```python
from build123d import *

# Parameters (mm, degrees)
SKETCH_1_R               = 20.5
EXTRUDE_1_DEPTH          = 5
HOLE_WIZARD_M5_1_D       = 5.3
HOLE_WIZARD_M5_2_D       = 5.3
HOLE_WIZARD_M5_2_DEPTH   = 5
CUT_EXTRUDE_1_DEPTH      = 2.5
HOLE_WIZARD_2_0_2_1_D    = 2
PATTERN_CIRCULAR_1_COUNT = 2


with BuildPart() as part:
    # 스케치1 → 보스-돌출1 (new, symmetric)
    with BuildSketch(Plane.XY):
        Circle(SKETCH_1_R)
    extrude(amount=EXTRUDE_1_DEPTH, both=True)

    # M5 여유 구멍1 (through all)
    with Locations(Plane.XY.offset(5)):
        with Locations((0, 0)):
            Hole(HOLE_WIZARD_M5_1_D / 2)

    # M5 여유 구멍2
    with Locations(Plane(origin=(0, 0, -5), x_dir=(-1, 0, 0), z_dir=(0, 0, -1))):
        with Locations((12.5, 0)):
            hole_wizard_m5_2 = Hole(HOLE_WIZARD_M5_2_D / 2, depth=HOLE_WIZARD_M5_2_DEPTH)

    # 대칭 복사1: M5 여유 구멍2 across plane
    add(hole_wizard_m5_2.mirror(Plane(origin=(0, 0, 0), x_dir=(0, 0, 1), z_dir=(1, 0, 0))), mode=Mode.SUBTRACT)

    # 스케치6 → 컷-돌출1 (cut)
    with BuildSketch(Plane.XY.offset(5)):
        with BuildLine():
            ThreePointArc((7.778174593, 7.778174593), (0, 11), (-7.778174593, 7.778174593))
            ThreePointArc((-7.778174593, 7.778174593), (-7.778174593, 3.535533906), (-3.535533906, 3.535533906))
            ThreePointArc((-3.535533906, 3.535533906), (0, 5), (3.535533906, 3.535533906))
            ThreePointArc((3.535533906, 3.535533906), (7.778174593, 3.535533906), (7.778174593, 7.778174593))
        make_face()
    cut_extrude_1 = extrude(amount=-CUT_EXTRUDE_1_DEPTH, mode=Mode.SUBTRACT)

    # Ø2.0 (2) 지름 구멍1 (through all)
    with Locations(Plane.XY.offset(2.5)):
        with Locations((0, 8)):
            hole_wizard_2_0_2_1 = Hole(HOLE_WIZARD_2_0_2_1_D / 2)

    # 원형 패턴1: 컷-돌출1, Ø2.0 (2) 지름 구멍1 ×2 about axis
    pattern_circular_1_axis = Axis((0, 0, 0), (0, 0, 1))
    add([cut_extrude_1.rotate(pattern_circular_1_axis, i * 360 / PATTERN_CIRCULAR_1_COUNT) for i in range(1, PATTERN_CIRCULAR_1_COUNT)], mode=Mode.SUBTRACT)
    add([hole_wizard_2_0_2_1.rotate(pattern_circular_1_axis, i * 360 / PATTERN_CIRCULAR_1_COUNT) for i in range(1, PATTERN_CIRCULAR_1_COUNT)], mode=Mode.SUBTRACT)


solid = part.part
```
The model under review builds one solid part; all positions refer to its coordinate system, in mm. A direction names the side the tool comes from. Round coordinates to 2 decimals unless told otherwise and drop trailing zeros. Order: outer loops, then holes, each group sorted by start corner. A loop starts at its lowest first (then second) coordinate and runs counter-clockwise, first axis right, second up. Notation, with made-up numbers: M 25.5,88 L 36.5,88 A19 cw 36.5,106 Z; hole C 13,0.5 d9. An arc over 180 degrees is marked long. Use a Markdown table: item, result.
1) Consider section B-B (z = -3.75). Write out the cut boundary in (x, y), then the cut area to 3 significant figures.
Report:
| item | result |
|---|---|
| outline | C 0,0 d41; hole C -12.5,0 d5.3; hole C 0,0 d5.3; hole C 0,-8 d2; hole C 0,8 d2; hole C 12.5,0 d5.3 |
| area | 1,250 mm^2 |
2) Consider section A-A (x = 0). Write out the cut boundary in (y, z).
Report:
| item | result |
|---|---|
| outline | M -20.5,-5 L -9,-5 L -9,2.5 L -11,2.5 L -11,5 L -20.5,5 Z; M -7,-5 L -2.65,-5 L -2.65,5 L -5,5 L -5,2.5 L -7,2.5 Z; M 2.65,-5 L 7,-5 L 7,2.5 L 5,2.5 L 5,5 L 2.65,5 Z; M 9,-5 L 20.5,-5 L 20.5,5 L 11,5 L 11,2.5 L 9,2.5 Z |
3) Wall thickness on line 1 along Y through (x, z) = (0, -2); line 2 along Y through (x, z) = (-7.5, 4); line 3 along Z through (x, y) = (-7, -6.5): over which ranges is each line inside the solid? List them lowest first. Write a range as [from, to].
Report:
| item | result |
|---|---|
| line 1 | [-20.5, -9], [-7, -2.65], [2.65, 7], [9, 20.5] |
| line 2 | [-19.08, -8.05], [-3.29, 3.29], [8.05, 19.08] |
| line 3 | [-5, 2.5] |
4) Insertion check: pin 1 (2.5 mm diameter, centred on x = -13.5, y = -0.5, fed in from -Z); pin 2 (6 mm diameter, centred on y = -11.5, z = 1.5, fed in from +X); pin 3 (1 mm diameter, centred on x = 7.5, z = -1, fed in from -Y); pin 4 (5 mm diameter, centred on x = 0, y = 0, fed in from -Z). Each pin has a flat end and moves straight along its axis. Give the tip position at first contact, or say it passes through.
Report:
| item | result |
|---|---|
| pin 1 | z = 0 |
| pin 2 | x = 18.65 |
| pin 3 | y = -19.27 |
| pin 4 | through |
5) Tool access review of faces 1 (the face through (-10.05, -1.01, -2.46)), 2 (the face through (0, -5, 4)), 3 (the face through (0, -9, -1)): name each direction out of +Z, -Z, +X, -X, +Y, -Y from which nothing blocks a thin tool from reaching the whole face with its end or side.
Report:
| item | result |
|---|---|
| face 1 | -Z |
| face 2 | +Z |
| face 3 | +Z, -Z |
6) Draft analysis for pull direction Y (two halves, no side actions). For faces 4 (the face through (13, 0, 0)), 5 (the face through (-4.444, -20.013, 0.07)), 6 (the face through (4, 0, -5)), state which applies: released by +Y, released by -Y, zero draft, split by the parting line, or undercut.
Report:
| item | result |
|---|---|
| face 4 | undercut |
| face 5 | split by the parting line |
| face 6 | zero draft |
7) Consider section C-C (y = -2). Write out the cut boundary in (x, z).
Report:
| item | result |
|---|---|
| outline | M -20.4,-5 L -14.24,-5 L -14.24,0 L -10.76,0 L -10.76,-5 L -1.74,-5 L -1.74,5 L -20.4,5 Z; M 1.74,-5 L 10.76,-5 L 10.76,0 L 14.24,0 L 14.24,-5 L 20.4,-5 L 20.4,5 L 1.74,5 Z |
8) Consider section D-D (z = 3.25). Write out the cut boundary in (x, y).
Report:
| item | result |
|---|---|
| outline | C 0,0 d41; hole M -7.78,-7.78 A11 ccw 7.78,-7.78 A3 ccw 3.54,-3.54 A5 cw -3.54,-3.54 A3 ccw Z; hole M -7.78,7.78 A3 ccw -3.54,3.54 A5 cw 3.54,3.54 A3 ccw 7.78,7.78 A11 ccw Z; hole C 0,0 d5.3 |
